Source: three-view drawing plus pictorial views. Frame: mm from the lowest corner of the part. A direction names the side the tool comes from. Give positions to 0.01 mm unless a question says otherwise; leave off trailing zeros. Loops run counter-clockwise (first coordinate to the right, second up) from the corner with the lowest first, then second, coordinate; pieces in that order, holes last. Notation, with made-up numbers: M 28.5,-34.5 L 53.5,-34.5 A16 ccw 53.5,-3.5 Z; hole C -24.75,60.25 d3. An arc over 180 degrees is marked long. Write item = value, one per line.
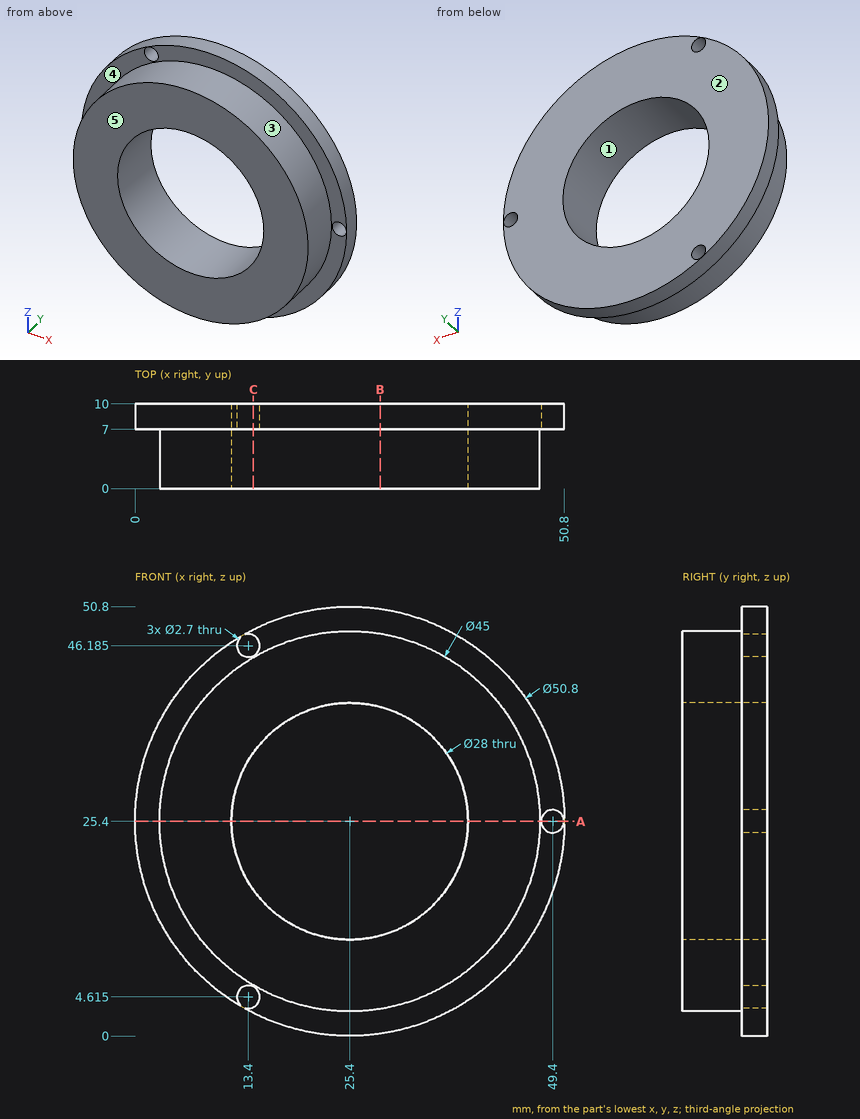
1. Cut plane B-B, the plane x = 29. Return the cut outline in (y, z), then the cut area to 3 significant figures.
Derived:
outline = M 0,3.19 L 7,3.19 L 7,0.26 L 10,0.26 L 10,11.87 L 0,11.87 Z; M 0,38.93 L 10,38.93 L 10,50.54 L 7,50.54 L 7,47.61 L 0,47.61 Z
area = 191 mm²
2. First-contact query: pin 1 Ø1.5 at (y, z) = (3.5, 39) entering from -X; pin 2 Ø17 at (x, z) = (25.4, 25.4) entering from -Y; pin 3 Ø5 at (y, z) = (7, 16) entering from -X (1 decimal); pin 4 Ø6 at (x, y) = (24, 4.5) entering from -Z. Flat tips, straight axial feed; report the tip coordinate or a pass-through.
Derived:
pin_1 = 6.93
pin_2 = through
pin_3 = 1
pin_4 = 0
3. Cut plane A-A, the plane z = 25.4. Return the cut outline in (x, y).
Derived:
outline = M 0,7 L 2.9,7 L 2.9,0 L 11.4,0 L 11.4,10 L 0,10 Z; M 39.4,0 L 47.9,0 L 47.9,7 L 48.05,7 L 48.05,10 L 39.4,10 Z; M 50.75,7 L 50.8,7 L 50.8,10 L 50.75,10 Z
4. Material intervals for probe 1 along Z at (x, y) = (13.4, 7.65) (1 decimal); probe 2 along Z at (x, y) = (14, 7.5) (1 decimal); probe 3 along X at (y, z) = (2.5, 25.4), sorted ascending. Write a range as from..to.
Derived:
probe_1 = 3..3.3, 6..18.2, 32.6..44.8, 47.5..47.8
probe_2 = 2.7..3.4, 5.8..17.3, 33.5..45, 47.4..48.1
probe_3 = 2.9..11.4, 39.4..47.9
5. Pull-direction query (Z, two-part tool) for the marked faces 1, 2 and 3; classes: +Z half, -Z half, draft (parallel to the pull), parting line (faces both ways), or undercut.
Derived:
face_1 = undercut
face_2 = draft
face_3 = parting line
6. Reachability of the marked faces 4 and 5 from +Z, -Z, +X, -X, +Y, -Y: full face, straight path, thin tool, end or side. Return the list, or none.
Derived:
face_4 = -Y
face_5 = +Z, -Z, +X, -X, -Y
7. Cut plane C-C, the plane x = 14. Count the separate pieces of the cut face and the enclosed holes in it, then the cut area to 3 significant figures.
Derived:
separate_pieces = 4
enclosed_holes = 0
area = 231 mm²
